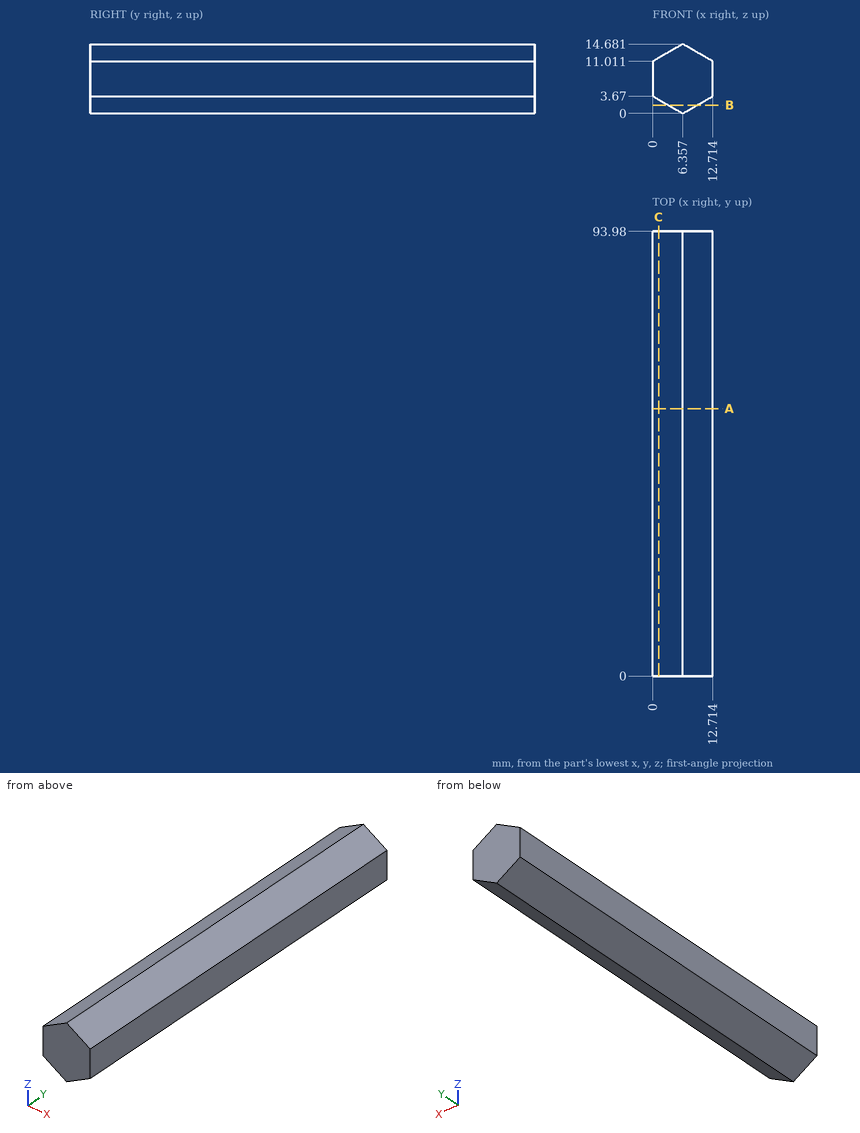
Drawing for the job (mm, zero at the part's lowest x, y, z). Give positions to 0.01 mm unless a question says otherwise; leave off trailing zeros. Loops run counter-clockwise (first coordinate to the right, second up) from the corner with the lowest first, then second, coordinate; pieces in that order, holes last.
(1) Drill centre lines: line 1 along Z through (x, y) = (1.25, 29); line 2 along Z through (x, y) = (10, 19.5); line 3 along X through (y, z) = (32.5, 14.25) (1 decimal). Where is each one in solid material? Low to high.
Return value:
line 1: z = 2.95 to 11.73
line 2: z = 2.1 to 12.58
line 3: x = 5.6 to 7.1
(2) Band-saw the part on A-A (y = 56.5). Write the cut outline in (x, z), and give its area (3 significant figures).
Return value:
outline: (0, 3.67) - (6.36, 0) - (12.71, 3.67) - (12.71, 11.01) - (6.36, 14.68) - (0, 11.01) - close
area: 140 mm2
(3) Pin check, flat tips, straight feed: pin 1 (2 mm diameter, centred on x = 9, y = 14.5, fed in from -Z); pin 2 (4 mm diameter, centred on x = 7.5, y = 61.5, fed in from +Z); pin 3 (6 mm diameter, centred on x = 7, y = 80, fed in from -Z). Stop position of each tip, or through.
Return value:
pin 1: stops at z = 0.95
pin 2: stops at z = 14.68
pin 3: stops at z = 0
(4) Band-saw the part on C-C (x = 1.25). Write the cut outline in (y, z).
Return value:
outline: (0, 2.95) - (93.98, 2.95) - (93.98, 11.73) - (0, 11.73) - close
(5) Band-saw the part on B-B (z = 1.75). Write the cut outline in (x, y).
Return value:
outline: (3.33, 0) - (9.39, 0) - (9.39, 93.98) - (3.33, 93.98) - close
